The listing builds one solid part. Answer for the finished solid, in the listing's coordinates (mm). Face numbers are marked on the shaded views. A direction names the side the tool comes from. Coordinates: 2 decimals unless noted, no trailing zeros. Write each loop counter-clockwise with the first axis right and the second up, starting at its lowest first coordinate (ties: lowest second). Pieces come first, ordered by that corner, then holes. Notation, with made-up numbers: M -13.5,17 L 25.5,17 A17 cw 25.5,37 Z; hole C 23,-34 d4. An arc over 180 degrees is marked long. Answer as CSV lines item,"result".
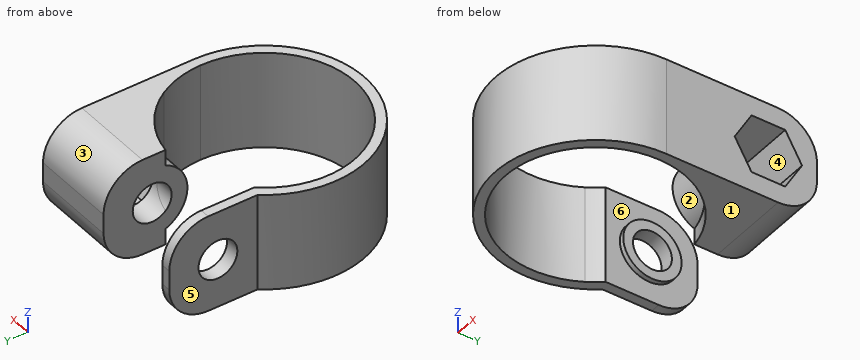
```python
from build123d import *

# Parameters (mm, degrees)
F1_DEPTH = 20
F2_R     = 4
F3_DEPTH = 40
F2_R_2   = 6
F4_DEPTH = 3
F5_R     = 7.25
F5_R_2   = 4
F6_DEPTH = 17.5
F7_DEPTH = 12
F8_R     = 8


# Not quite as in the source:
# - a feature names something its author has since deleted; it is built from what else it names


with BuildPart() as f1:
    # F0 (on Top) → F1 (new body)
    with BuildSketch(Plane.XY):
        with BuildLine():
            Line((20.5, 0), (18.5, 0))
            ThreePointArc((18.5, 0), (-4.8088460154, -17.8640700849), (-16, 9.2870878105))
            Line((-16, 9.2870878105), (-16, 12.816005618))
            ThreePointArc((-16, 12.816005618), (-6.7915388536, -19.3423111339), (20.5, 0))
        make_face()
        with BuildLine():
            Line((-16, 31), (-16, 12.816005618))
            ThreePointArc((-16, 12.816005618), (-15.0387928923, 13.9314287976), (-14, 14.9749791319))
            Line((-14, 14.9749791319), (-14, 31))
            Line((-14, 31), (-16, 31))
        make_face()
        with BuildLine():
            Line((-16, 12.816005618), (-16, 9.2870878105))
            ThreePointArc((-16, 9.2870878105), (-15.0654846671, 10.7369069915), (-14, 12.0933866224))
            Line((-14, 12.0933866224), (-14, 14.9749791319))
            ThreePointArc((-14, 14.9749791319), (-15.0387928923, 13.9314287976), (-16, 12.816005618))
        make_face()
        with BuildLine():
            ThreePointArc((16, 12.816005618), (19.3423111339, 6.7915388536), (20.5, 0))
            Line((20.5, 0), (20.5, 31))
            Line((20.5, 31), (16, 31))
            Line((16, 31), (16, 12.816005618))
        make_face()
        with BuildLine():
            ThreePointArc((16, 9.2870878105), (17.8640700849, 4.8088460154), (18.5, 0))
            Line((18.5, 0), (20.5, 0))
            ThreePointArc((20.5, 0), (19.3423111339, 6.7915388536), (16, 12.816005618))
            Line((16, 12.816005618), (16, 9.2870878105))
        make_face()
        with BuildLine():
            ThreePointArc((3, 20.2792997907), (10.2066248083, 17.7784929064), (16, 12.816005618))
            Line((16, 12.816005618), (16, 31))
            Line((16, 31), (3, 31))
            Line((3, 31), (3, 20.2792997907))
        make_face()
        with BuildLine():
            ThreePointArc((3, 18.2551362635), (10.5050689319, 15.2280506545), (16, 9.2870878105))
            Line((16, 9.2870878105), (16, 12.816005618))
            ThreePointArc((16, 12.816005618), (10.2066248083, 17.7784929064), (3, 20.2792997907))
            Line((3, 20.2792997907), (3, 18.2551362635))
        make_face()
    extrude(amount=F1_DEPTH)

    # F2 (on face) → F3 (cut)
    with BuildSketch(Plane(origin=(-16, 0, 0), x_dir=(0, -1, 0), z_dir=(-1, 0, 0))):
        with Locations((-21, 10)):
            Circle(F2_R)
    extrude(amount=-F3_DEPTH, mode=Mode.SUBTRACT)

    # F2 (on face) → F4 (join)
    with BuildSketch(Plane(origin=(-16, 0, 0), x_dir=(0, -1, 0), z_dir=(-1, 0, 0))):
        with Locations((-21, 10)):
            Circle(F2_R_2)
        with Locations((-21, 10)):
            Circle(F2_R, mode=Mode.SUBTRACT)
    extrude(amount=-F4_DEPTH)

    # F5 (on face) → F6 (join)
    with BuildSketch(Plane.YZ.offset(20.5)):
        with Locations((21, 10)):
            Circle(F5_R)
        Polygon((14.0717967697, 10), (17.5358983849, 16), (24.4641016151, 16), (27.9282032303, 10), (24.4641016151, 4), (17.5358983849, 4), align=None, mode=Mode.SUBTRACT)
        Polygon((24.4641016151, 16), (17.5358983849, 16), (14.0717967697, 10), (17.5358983849, 4), (24.4641016151, 4), (27.9282032303, 10), align=None)
        with Locations((21, 10)):
            Circle(F5_R_2, mode=Mode.SUBTRACT)
    extrude(amount=-F6_DEPTH)

    # F5 (on face) → F7 (cut)
    with BuildSketch(Plane.YZ.offset(20.5)):
        Polygon((24.4641016151, 16), (17.5358983849, 16), (14.0717967697, 10), (17.5358983849, 4), (24.4641016151, 4), (27.9282032303, 10), align=None)
        with Locations((21, 10)):
            Circle(F5_R_2, mode=Mode.SUBTRACT)
    extrude(amount=-F7_DEPTH, mode=Mode.SUBTRACT)

    # F8
    f8_edges = [f1.edges().sort_by_distance(p)[0] for p in [
        (11.75, 31, 20),
        (-15, 31, 20),
        (11.75, 31, 0),
        (-15, 31, 0),
    ]]
    fillet(f8_edges, radius=F8_R)


solid = f1.part
```
Q1. For the marked faces 4, 5 and 6, determine the directions among +Z, -Z, +X, -X, +Y, -Y from which every point of the face is accessible in a straight line to the end or side of a thin tool.
Output:
face 4,"+X"
face 5,"+Z, -Z, -X, +Y"
face 6,"none"
Q2. The mould has two halves that part along Y. Classify the marked faces 1, 2 and 3: pulls with the +Y half, pulls with the -Y half, needs draft (parallel to the pull), parting line crosses it, or undercut.
Output:
face 1,"needs draft"
face 2,"undercut"
face 3,"pulls with the +Y half"
Q3. Find section A-A (x = 14). Give the vertices of the cut face in (y, z).
Output:
outline,"M -14.97,0 L -12.09,0 L -12.09,20 L -14.97,20 Z; M 12.09,0 L 23,0 A8 ccw 31,8 L 31,12 A8 ccw 23,20 L 12.09,20 Z; hole M 14.07,10 L 17.54,4 L 24.46,4 L 27.93,10 L 24.46,16 L 17.54,16 Z"
Q4. Straight lines are drawn through the part: line 1 (Y direction, x = 10, z = 14.5); line 2 (Y direction, x = 5.05, z = 10); line 3 (Z direction, x = -14.85, y = 21). For each, find the intervals that lie inside material, in ascending order.
Output:
line 1,"-17.9 to -15.56, 15.32 to 16.67, 25.33 to 30.6"
line 2,"-19.87 to -17.8, 13.75 to 17, 25 to 31"
line 3,"0 to 6, 14 to 20"
Q5. Flat-ended cylindrical pins translate along their axes: pin 1 Ø5 at (x, z) = (-3, 18) entering from +Y; pin 2 Ø8.5 at (y, z) = (19.5, 12) entering from -X; pin 3 Ø5 at (x, z) = (-14, 5) entering from -Y. Find the tip coordinate at first contact, or state that the pin passes through.
Output:
pin 1,"y = -17.66"
pin 2,"x = -16"
pin 3,"y = -16.97"
Q6. Find section C-C (x = 6). Give the vertices of the cut face in (y, z).
Output:
outline,"M -19.6,0 L -17.5,0 L -17.5,20 L -19.6,20 Z; M 17.5,0 L 23,0 A8 ccw 31,8 L 31,12 A8 ccw 23,20 L 17.5,20 L 17.5,16.35 A7.25 ccw 17.5,3.65 Z; hole C 21,10 d8"
Q7. Find section B-B (y = -11.5). Give the vertices of the cut face in (x, z), and give its area (3 significant figures).
Output:
outline,"M -16.97,0 L -14.49,0 L -14.49,20 L -16.97,20 Z; M 14.49,0 L 16.97,0 L 16.97,20 L 14.49,20 Z"
area,"99.2 mm2"
Q8. Find section D-D (z = 17.5). Give the vertices of the cut face in (x, y).
Output:
outline,"M -16,12.82 A20.5 ccw long 20.5,0 L 20.5,28.81 L 3,28.81 L 3,18.26 A18.5 cw long -14,12.09 L -14,28.81 L -16,28.81 Z"
